```python
from build123d import *

# Parameters (mm, degrees)
BOSS_EXTRUDE1_DEPTH      = 50
BOSS_EXTRUDE1_DEPTH_BACK = 50
CUT_EXTRUDE2_DEPTH       = 198.230829233
CUT_EXTRUDE2_DEPTH_BACK  = 15
BOSS_EXTRUDE2_DEPTH      = 25
BOSS_EXTRUDE2_DEPTH_BACK = 25
SKETCH8_R                = 10
CUT_EXTRUDE3_DEPTH       = 170.115345253
CUT_EXTRUDE5_REACH       = 179.2
SKETCH11_W               = 30
SKETCH11_H               = 20
CUT_EXTRUDE8_REACH       = 179.2
SKETCH14_W               = 40
SKETCH14_H               = 15


with BuildPart() as part:
    # Sketch1 → Boss-Extrude1 (new, two sides: drawn at the far end of the back side and taken through both)
    with BuildSketch(Plane.XY.offset(-BOSS_EXTRUDE1_DEPTH_BACK)):
        Polygon((0, 0), (0, 80), (30, 80), (150, 20), (150, 0), align=None)
    extrude(amount=BOSS_EXTRUDE1_DEPTH + BOSS_EXTRUDE1_DEPTH_BACK)

    # Sketch6 → Cut-Extrude2 (cut, two sides: drawn at the far end of the back side and taken through both)
    with BuildSketch(Plane.XY.offset(50).offset(-CUT_EXTRUDE2_DEPTH_BACK)):
        with BuildLine():
            Line((-326.513861399, 50.45053136), (0, 50.45053136))
            ThreePointArc((0, 50.45053136), (35.673912839, 35.673912839), (50.45053136, 0))
            Line((50.45053136, 0), (50.45053136, -326.513861399))
            Line((50.45053136, -326.513861399), (-411.309799734, -788.274192493))
            Line((-411.309799734, -788.274192493), (-788.274192493, -411.309799734))
            Line((-788.274192493, -411.309799734), (-326.513861399, 50.45053136))
        make_face()
    extrude(amount=CUT_EXTRUDE2_DEPTH + CUT_EXTRUDE2_DEPTH_BACK, mode=Mode.SUBTRACT)

    # Sketch7 → Boss-Extrude2 (add, two sides: drawn at the far end of the back side and taken through both)
    with BuildSketch(Plane.XY.offset(-BOSS_EXTRUDE2_DEPTH_BACK)):
        Polygon((70, 60), (130, 60), (130, 30), align=None)
    extrude(amount=BOSS_EXTRUDE2_DEPTH + BOSS_EXTRUDE2_DEPTH_BACK)

    # Sketch8 → Cut-Extrude3 (cut, through all)
    with BuildSketch(Plane(origin=(0, 60, 0), x_dir=(1, 0, 0), z_dir=(0, 1, 0))):
        with Locations(Location((100, 0, 0), (0, 0, 270))):
            Circle(SKETCH8_R)
    extrude(amount=-CUT_EXTRUDE3_DEPTH, mode=Mode.SUBTRACT)

    # Cut-Extrude5: up to this plane
    cut_extrude5_end = Plane(origin=(30, 80, 50), z_dir=(-0.447213595499958, -0.894427190999916, 0))
    # Sketch11 → Cut-Extrude5 (cut, up to the surface)
    with BuildSketch(Plane(origin=(0, 0, 0), x_dir=(0, 0, -1), z_dir=(1, 0, 0)), mode=Mode.PRIVATE) as cut_extrude5_sk1:
        with Locations((0, 70)):
            Rectangle(SKETCH11_W, SKETCH11_H)
    cut_extrude5_tool1 = split(extrude(cut_extrude5_sk1.sketch, amount=CUT_EXTRUDE5_REACH, mode=Mode.PRIVATE), bisect_by=cut_extrude5_end, keep=Keep.BOTH, mode=Mode.PRIVATE)
    add(cut_extrude5_tool1.solids().sort_by_distance((0, 70, 0))[0], mode=Mode.SUBTRACT)

    # Cut-Extrude8: up to this plane
    cut_extrude8_end = Plane(origin=(30, 80, 50), z_dir=(-0.447213595499958, -0.894427190999916, 0))
    # Sketch14 → Cut-Extrude8 (cut, up to the surface)
    with BuildSketch(Plane.XZ, mode=Mode.PRIVATE) as cut_extrude8_sk1:
        with Locations((100, 42.5)):
            Rectangle(SKETCH14_W, SKETCH14_H)
    cut_extrude8_tool1 = split(extrude(cut_extrude8_sk1.sketch, amount=-CUT_EXTRUDE8_REACH, mode=Mode.PRIVATE), bisect_by=cut_extrude8_end, keep=Keep.BOTH, mode=Mode.PRIVATE)
    add(cut_extrude8_tool1.solids().sort_by_distance((100, 0, 42.5))[0], mode=Mode.SUBTRACT)


solid = part.part
```
CAD build for the part. Positions are in the model's coordinates, mm. A direction names the side the tool comes from. Round coordinates to 2 decimals unless told otherwise and drop trailing zeros. Order: outer loops, then holes, each group sorted by start corner. A loop starts at its lowest first (then second) coordinate and runs counter-clockwise, first axis right, second up.
Item 1: Saw through at B-B on x = 100. Write the cut outline in (y, z), then the cut area to 4 significant figures.
Item 2: Mould opens along Z. For faces 4 (the face through (27, 68, -15)), 5 (the face through (59, 32, -50)), 6 (the face through (150, 10, -1)) say: pulls with the +Z half, pulls with the -Z half, needs draft (parallel to the pull), parting line crosses it, or undercut.
Item 3: Saw through at D-D on z = 0. Write the cut outline in (x, y), then the cut area to 3 significant figures.
Item 4: Probe line 1 along Z through (x, y) = (40, 73); line 2 along X through (y, z) = (40, 0); line 3 along Y through (x, z) = (114.5, 7.5). List the from-to ranges inside material, lowest first.
Item 5: Saw through at A-A on z = 40.5. Write the cut outline in (x, y), then the cut area to 3 significant figures.
Item 6: Tool access for faces 1 (the face through (35.28, 36.064, 42.395)), 2 (the face through (107, 49, 25)), 3 (the face through (120, 17, 42)): list every direction of +Z, -Z, +X, -X, +Y, -Y with a clear straight run to the whole face (end or side of a thin tool).
Item 7: Pin check, flat tips, straight feed: pin 1 (15 mm diameter, centred on x = 104.5, y = 51.5, fed in from -Z); pin 2 (7.5 mm diameter, centred on y = 13, z = 41, fed in from -X); pin 3 (9 mm diameter, centred on y = 42, z = -7, fed in from +X). Stop position of each tip, or through.
Item 8: Saw through at C-C on y = 5. Write the cut outline in (x, z).
Reported:
1. outline: (0, -50) - (45, -50) - (45, -25) - (60, -25) - (60, -10) - (0, -10) - close; (0, 10) - (60, 10) - (60, 25) - (45, 25) - (45, 35) - (0, 35) - close
1. area: 3,375 mm2
2. face 4: undercut
2. face 5: pulls with the -Z half
2. face 6: needs draft
3. outline: (0, 0) - (90, 0) - (90, 60) - (0, 60) - close; (110, 0) - (150, 0) - (150, 20) - (130, 30) - (130, 60) - (110, 60) - close
3. area: 7,100 mm2
4. line 1: z = -50 to -15, 15 to 50
4. line 2: x = 0 to 90, 110 to 130
4. line 3: y = 0 to 60
5. outline: (0, 50.45) arc R50.45 cw to (50.45, 0) - (80, 0) - (80, 55) - (30, 80) - (0, 80) - close; (120, 0) - (150, 0) - (150, 20) - (120, 35) - close
5. area: 4,600 mm2
6. face 1: +Z, -X, -Y
6. face 2: +Z, +X, +Y
6. face 3: +Z, +Y, -Y
7. pin 1: stops at z = -25
7. pin 2: stops at x = 47.59
7. pin 3: stops at x = 130
8. outline: (0, -50) - (150, -50) - (150, 50) - (120, 50) - (120, 35) - (80, 35) - (80, 50) - (50.2, 50) - (50.2, 35) - (0, 35) - close; hole circle Ø20 at (100, 0)
